Read the model definition and answer for the solid it produces. Units are mm, in the model's axes. Coordinates: 2 decimals unless noted, no trailing zeros. Order: outer loops, then holes, each group sorted by start corner. A loop starts at its lowest first (then second) coordinate and runs counter-clockwise, first axis right, second up. Notation, with made-up numbers: (51.25, 18) -> (70.25, 18) arc R30 cw to (70.25, 55) -> close; hole circle Ø10 at (41, 27.5). An arc over 180 degrees is marked (long way). Use CSV: the item, a comma, the result in double quotes.
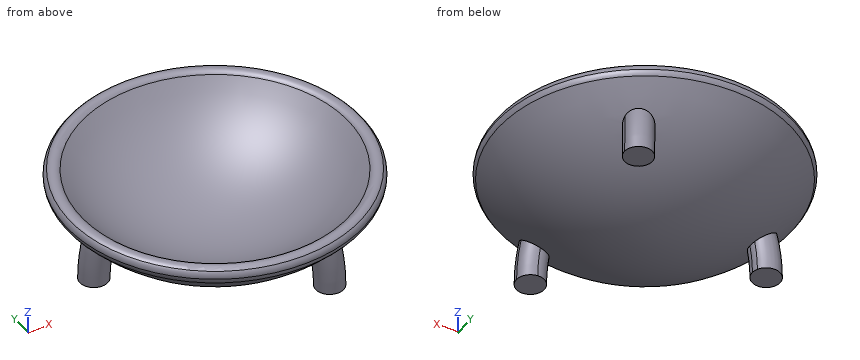
```python
from build123d import *

# Parameters (mm, degrees)
F3_ANGLE = 15
F4_ANGLE = 15
F5_ANGLE = 15


with BuildPart() as f2:
    # F1 (on Right) → F2 (revolve)
    with BuildSketch(Plane.YZ):
        with BuildLine():
            ThreePointArc((-23.5, 12.700896879), (-23.6243333512, 12.1029493301), (-23.9767216951, 11.6041282112))
            ThreePointArc((-23.9767216951, 11.6041282112), (-13.0093869009, 4.1292071294), (0, 1.5))
            Line((0, 1.5), (0, 3))
            ThreePointArc((0, 3), (-13.0839530364, 5.7970862251), (-23.8805970223, 13.6993641912))
            ThreePointArc((-23.8805970223, 13.6993641912), (-23.5983751453, 13.235169999), (-23.5, 12.700896879))
        make_face()
        with BuildLine():
            ThreePointArc((-23.9767216951, 11.6041282112), (-25.0687443502, 11.2024729689), (-26.119403059, 11.7024296579))
            ThreePointArc((-26.119403059, 11.7024296579), (-14.3105736787, 3.059313079), (0, 0))
            Line((0, 0), (0, 1.5))
            ThreePointArc((0, 1.5), (-13.0093869009, 4.1292071294), (-23.9767216951, 11.6041282112))
        make_face()
        with BuildLine():
            ThreePointArc((-25.9731557832, 13.842373038), (-26.4965092865, 12.8031708029), (-26.119403059, 11.7024296579))
            ThreePointArc((-26.119403059, 11.7024296579), (-25.0687443502, 11.2024729689), (-23.9767216951, 11.6041282112))
            ThreePointArc((-23.9767216951, 11.6041282112), (-25, 12.700896879), (-25.9731557832, 13.842373038))
        make_face()
        with BuildLine():
            ThreePointArc((-23.8805970223, 13.6993641912), (-24.897726137, 14.1974061697), (-25.9731557832, 13.842373038))
            ThreePointArc((-25.9731557832, 13.842373038), (-25, 12.700896879), (-23.9767216951, 11.6041282112))
            ThreePointArc((-23.9767216951, 11.6041282112), (-23.6243333512, 12.1029493301), (-23.5, 12.700896879))
            ThreePointArc((-23.5, 12.700896879), (-23.5983751453, 13.235169999), (-23.8805970223, 13.6993641912))
        make_face()
        with BuildLine():
            ThreePointArc((23.9767216951, 11.6041282112), (25.0687443844, 11.2024729705), (26.1194031045, 11.702429709))
            ThreePointArc((26.1194031045, 11.702429709), (26.4016248886, 12.166623848), (26.5, 12.700896879))
            ThreePointArc((26.5, 12.700896879), (26.3619349608, 13.3294930631), (25.9731557832, 13.842373038))
            ThreePointArc((25.9731557832, 13.842373038), (25, 12.700896879), (23.9767216951, 11.6041282112))
        make_face()
        with BuildLine():
            ThreePointArc((23.8805969652, 13.6993641272), (23.5015760891, 12.6321525469), (23.9767216951, 11.6041282112))
            ThreePointArc((23.9767216951, 11.6041282112), (25, 12.700896879), (25.9731557832, 13.842373038))
            ThreePointArc((25.9731557832, 13.842373038), (24.8977260943, 14.1974061667), (23.8805969652, 13.6993641272))
        make_face()
    revolve(axis=Axis((0, 0, 69.2957118154), (0, 0, 1)))

    # F0 (on Top) → F3 (revolve)
    with BuildSketch(Plane.XY):
        with BuildLine():
            ThreePointArc((11.4392372684, -19.0023692486), (10.7795747302, -17.3102823634), (9.1487108469, -16.5111605419))
            Line((9.1487108469, -16.5111605419), (8.9392372684, -19.0023692486))
            Line((8.9392372684, -19.0023692486), (6.8865240316, -17.5753554549))
            ThreePointArc((6.8865240316, -17.5753554549), (8.1915017176, -21.3879282074), (11.4392372684, -19.0023692486))
        make_face()
        with BuildLine():
            Line((8.9392372684, -19.0023692486), (9.1487108469, -16.5111605419))
            ThreePointArc((9.1487108469, -16.5111605419), (7.8750423555, -16.7401824333), (6.8865240316, -17.5753554549))
            Line((6.8865240316, -17.5753554549), (8.9392372684, -19.0023692486))
        make_face()
    revolve(axis=Axis((-4.4696186342, 9.5011846243, 0), (-0.9048747261, -0.4256779652, 0)), revolution_arc=F3_ANGLE)

    # F0 (on Top) → F4 (revolve)
    with BuildSketch(Plane.XY):
        with BuildLine():
            Line((11.7774422886, 14.7515824826), (11.9869158671, 17.2427911892))
            Line((11.9869158671, 17.2427911892), (9.7247290518, 16.1785962763))
            ThreePointArc((9.7247290518, 16.1785962763), (10.5599020734, 15.1900779524), (11.7774422886, 14.7515824826))
        make_face()
        with BuildLine():
            Line((9.7247290518, 16.1785962763), (11.9869158671, 17.2427911892))
            Line((11.9869158671, 17.2427911892), (11.7774422886, 14.7515824826))
            ThreePointArc((11.7774422886, 14.7515824826), (13.6790027523, 15.4024537275), (14.4869158671, 17.2427911892))
            ThreePointArc((14.4869158671, 17.2427911892), (11.4416943701, 19.6826136252), (9.7247290518, 16.1785962763))
        make_face()
    revolve(axis=Axis((-5.9934579336, -8.6213955946, 0), (0.8210852947, -0.5708055175, 0)), revolution_arc=F4_ANGLE)

    # F0 (on Top) → F5 (revolve)
    with BuildSketch(Plane.XY):
        with BuildLine():
            ThreePointArc((-18.4261531356, 1.7595780594), (-18.4863306996, 2.3047995564), (-18.6639663203, 2.8237729723))
            Line((-18.6639663203, 2.8237729723), (-20.9261531356, 1.7595780594))
            Line((-20.9261531356, 1.7595780594), (-18.8734398988, 0.3325642656))
            ThreePointArc((-18.8734398988, 0.3325642656), (-18.5405941767, 1.0118425085), (-18.4261531356, 1.7595780594))
        make_face()
        with BuildLine():
            Line((-20.9261531356, 1.7595780594), (-18.6639663203, 2.8237729723))
            ThreePointArc((-18.6639663203, 2.8237729723), (-23.4173618422, 1.9690516378), (-18.8734398988, 0.3325642656))
            Line((-18.8734398988, 0.3325642656), (-20.9261531356, 1.7595780594))
        make_face()
    revolve(axis=Axis((10.4630765678, -0.8797890297, 0), (0.0837894314, 0.9964834826, 0)), revolution_arc=F5_ANGLE)


solid = f2.part
```
Item 1: Straight lines are drawn through the part: line 1 along X through (y, z) = (5.5, 13.75); line 2 along Y through (x, z) = (11, 9.75); line 3 along X through (y, z) = (2, 6.5). For each, find the intervals that lie inside material, in ascending order.
Return value:
line 1,"x = -25.49 to -23.29, 23.29 to 25.49"
line 2,"y = -21.6 to -16.29, 16.29 to 21.6"
line 3,"x = -22.78 to -14.41, 14.41 to 20.22"
Item 2: Each of these flat-tipped pins is pushed along its axis until it touches: P1, Ø6, axis at x = 5.5, y = -7, coming from the +Z side; P2, Ø8, axis at y = 15, z = 10.5, coming from the +X side; P3, Ø2, axis at x = 4, y = -19.5, coming from the -Z side. Where does it stop, or does it pass through?
Return value:
P1,"stops at z = 5.3"
P2,"stops at x = 23.85"
P3,"stops at z = 5.55"
Item 3: Find section B-B, the plane z = 9.25. Give the vertices of the cut face in (x, y), then the cut area to 3 significant figures.
Return value:
outline,"circle Ø47.41 at (0, 0); hole circle Ø38 at (0, 0)"
area,"631 mm^2"
